Autodesk Inventor part; units mm, degrees
ref_plane "YZ Plane" through (0, 0, 0) normal (1, 0, 0) x (0, 1, 0)
ref_plane "XZ Plane" through (0, 0, 0) normal (0, 1, 0) x (-1, 0, 0)
ref_plane "XY Plane" through (0, 0, 0) normal (0, 0, 1) x (1, 0, 0)
sketch "Sketch2" plane through (0, 0, 0) normal (0, 0, 1) x (1, 0, 0)
  line L0 (-75, -25) -> (75, -25)
  line L1 (75, -25) -> (75, 25)
  line L2 (75, 25) -> (-75, 25)
  line L3 (-75, 25) -> (-75, -25)
  line L4 (-75, -25) -> (75, 25) construction
  line L5 (75, -25) -> (-75, 25) construction
  point P0 (0, 0)
  dimension "d1" = 150
  dimension "d2" = 50
extrude "Extrusion1" add sketch "Sketch2" along normal mid plane 10
sketch "Sketch3" plane through (0, 0, 5) normal (0, 0, 1) x (1, 0, 0)
  line L0 (-75, 25) -> (-75, -25)
  line L1 (75, 25) -> (-75, 25)
  point P0 (0, 0)
  point P1 (-65, 0)
  dimension "d40" = 10
  dimension "d43" = 25
hole "Hole1" at (-65, 0, 5) direction (0, 0, -1) diameter 5.5 depth 14.2 tip angle 118 counterbore diameter 10 counterbore depth 5.4
sketch "Sketch4" plane through (0, 0, 5) normal (0, 0, 1) x (1, 0, 0)
  line L0 (-75, 25) -> (-75, -25)
  line L1 (75, 25) -> (-75, 25)
  point P0 (0, 0)
  point P1 (-45, 5)
  dimension "d41" = 30
  dimension "d42" = 20
hole "Hole2" at (-45, 5, 5) direction (0, 0, -1) diameter 6.6 depth 17.1 tip angle 118 counterbore diameter 11 counterbore depth 6.5
sketch "Sketch5" plane through (0, 0, 5) normal (0, 0, 1) x (1, 0, 0)
  line L0 (-75, 25) -> (-75, -25)
  line L1 (75, 25) -> (-75, 25)
  point P0 (0, 0)
  point P1 (-24, 10)
  dimension "d44" = 51
  dimension "d45" = 15
hole "Hole3" at (-24, 10, 5) direction (0, 0, -1) diameter 9 depth 22.2 tip angle 118 counterbore diameter 15 counterbore depth 8.6
sketch "Sketch6" plane through (0, 0, 5) normal (0, 0, 1) x (1, 0, 0)
  line L0 (-75, 25) -> (-75, -25)
  line L1 (75, 25) -> (-75, 25)
  point P0 (0, 0)
  point P1 (6, 5)
  dimension "d46" = 81
  dimension "d47" = 20
hole "Hole4" at (6, 5, 5) direction (0, 0, -1) diameter 6 depth 14.2 tip angle 118
sketch "Sketch7" plane through (0, 0, 5) normal (0, 0, 1) x (1, 0, 0)
  line L0 (-75, 25) -> (-75, -25)
  line L1 (75, 25) -> (-75, 25)
  point P0 (0, 0)
  point P1 (25, 10)
  dimension "d48" = 100
  dimension "d49" = 15
hole "Hole5" at (25, 10, 5) direction (0, 0, -1) diameter 10 depth 14.2 tip angle 118
pattern_linear "Rectangular Pattern1" count 3 spacing 10 along (0, -1, 0) of "Hole1" first direction both ways yes
mirror "Mirror1" about plane through (0, 0, 0) normal (0, 1, 0) of "Hole2"
mirror "Mirror2" about plane through (0, 0, 0) normal (0, 1, 0) of "Hole3"
pattern_linear "Rectangular Pattern2" count 3 spacing 10 along (0, -1, 0) of "Hole4"
mirror "Mirror3" about plane through (0, 0, 0) normal (0, 1, 0) of "Hole5"
properties part number "홀간 거리 확인 파트-12" material "SS400"
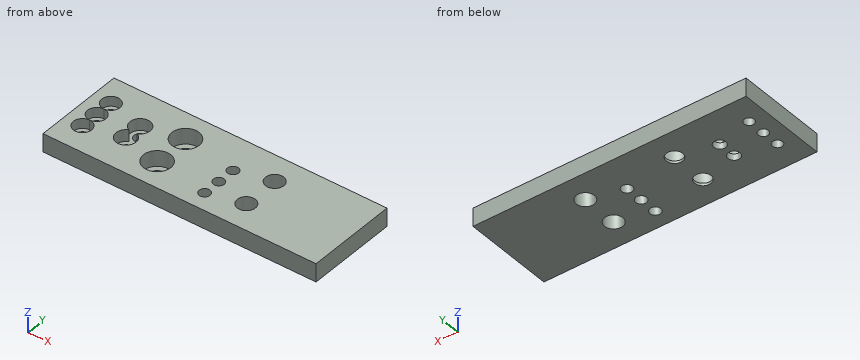
Input: part model. Units: mm. Frame: model coordinates. Give positions to 0.01 mm unless a question says otherwise; leave off trailing zeros. Loops run counter-clockwise (first coordinate to the right, second up) from the corner with the lowest first, then second, coordinate; pieces in that order, holes last.
1) Line query: L1, parallel to Y at x = -24, z = 2.5; L2, parallel to Y at x = -65, z = -1.95; L3, parallel to X at y = -10, z = -2.8. Output: solid intervals per line, ascending.
A:
L1: y = -25 to -17.5, -2.5 to 2.5, 17.5 to 25
L2: y = -25 to -12.75, -7.25 to -2.75, 2.75 to 7.25, 12.75 to 25
L3: x = -75 to -67.75, -62.25 to -31.5, -16.5 to 20, 30 to 75
2) Section query A-A on x = -45. Return the cut outline in (y, z).
A:
outline: (-25, -5) - (-8.3, -5) - (-8.3, -1.5) - (-10.5, -1.5) - (-10.5, 5) - (-25, 5) - close; (-1.7, -5) - (1.7, -5) - (1.7, -1.5) - (-1.7, -1.5) - close; (8.3, -5) - (25, -5) - (25, 5) - (10.5, 5) - (10.5, -1.5) - (8.3, -1.5) - close
3) Section query B-B on x = -24. Return the cut outline in (y, z).
A:
outline: (-25, -5) - (-14.5, -5) - (-14.5, -3.6) - (-17.5, -3.6) - (-17.5, 5) - (-25, 5) - close; (-5.5, -5) - (5.5, -5) - (5.5, -3.6) - (2.5, -3.6) - (2.5, 5) - (-2.5, 5) - (-2.5, -3.6) - (-5.5, -3.6) - close; (14.5, -5) - (25, -5) - (25, 5) - (17.5, 5) - (17.5, -3.6) - (14.5, -3.6) - close
4) Contact query for flat-ended pins moving along their axis: pin 1 (3.5 mm diameter, centred on x = 6, y = -5, fed in from +Z); pin 2 (6 mm diameter, centred on x = -65, y = 10, fed in from +Z); pin 3 (4.5 mm diameter, centred on x = -21, y = -8, fed in from +Z). Output: stop coordinate, or through.
A:
pin 1: passes through
pin 2: stops at z = -0.4
pin 3: stops at z = -3.6
